Could you check a few things on this drawing? It's one solid part, dimensions in mm from its lowest x, y, z. A direction names the side the tool comes from. Coordinates: 2 decimals unless noted, no trailing zeros. Order: outer loops, then holes, each group sorted by start corner. A loop starts at its lowest first (then second) coordinate and runs counter-clockwise, first axis right, second up.
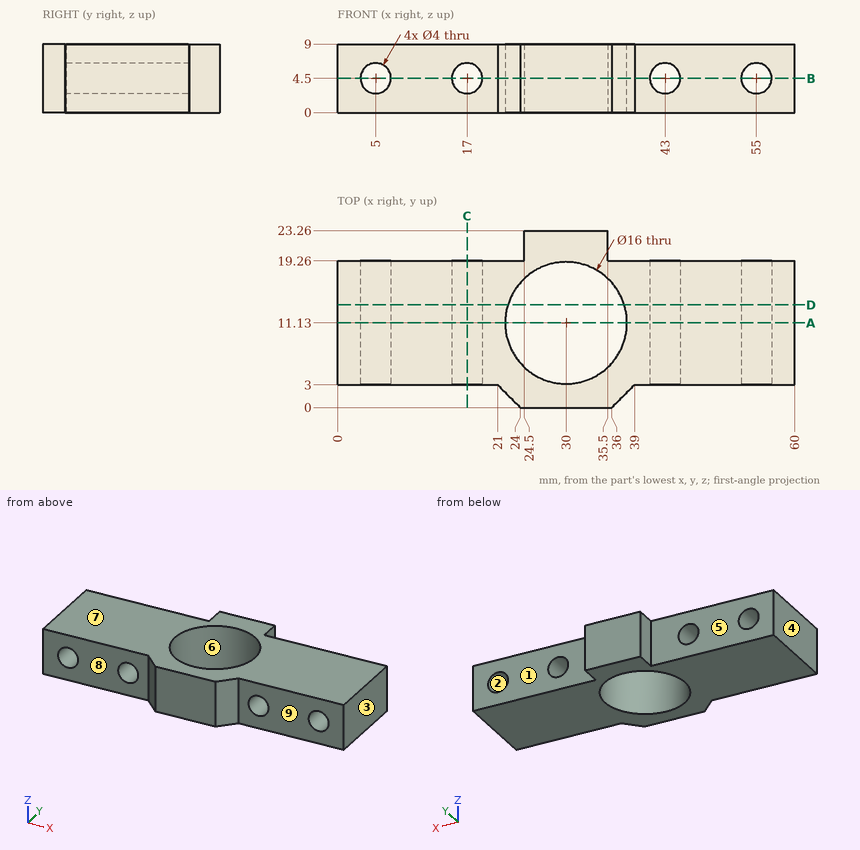
Item 1: Thinking about a two-plate mould opening in X: for the marked faces 1, 2, 3 and 4, which applies, +X half, -X half, draft (parallel to the pull), parting line (faces both ways), or undercut?
Item 2: For pin 1 Ø4 at (x, z) = (46.5, 1) entering from -Y; pin 2 Ø3 at (y, z) = (22.5, 4) entering from -X; pin 3 Ø3 at (y, z) = (21.5, 3) entering from +X; pin 4 Ø3 at (x, z) = (43, 4.5) entering from +Y, each with a flat end and sliding along its axis, tell me the tip position at first contact or that it passes through.
Item 3: Suppose I cut it at A-A (y = 11.13). List the corners of the cut face in (x, z) for me, and give its area (3 significant figures).
Item 4: Suppose I cut it at C-C (x = 17). List the corners of the cut face in (y, z) for me.
Item 5: Suppose I cut it at B-B (z = 4.5). Count the separate pieces of the cut face and the enclosed holes in it, and give its area (3 significant figures).
Item 6: Which directions (+Z, -Z, +X, -X, +Y, -Y) give clear straight access to the entire face, cutting with the end or side of a thin tool? Please do the marked faces 5, 6, 7, 8 and 9.
Item 7: I need wall thicknesses on line 1 (X direction, y = 11.25, z = 4.5); line 2 (X direction, y = 3.75, z = 2.75); line 3 (Y direction, x = 54.5, z = 1.75). Which ranges of each line are inside material? Lowest first, please.
Item 8: Suppose I cut it at D-D (y = 13.5). List the corners of the cut face in (x, z) for me, and give its area (3 significant figures).
Geometry results:
1. face 1: draft
1. face 2: undercut
1. face 3: +X half
1. face 4: -X half
2. pin 1: stops at y = 3
2. pin 2: stops at x = 24.5
2. pin 3: stops at x = 35.5
2. pin 4: passes through
3. outline: (0, 0) - (22, 0) - (22, 9) - (0, 9) - close; (38, 0) - (60, 0) - (60, 9) - (38, 9) - close; hole circle Ø4 at (5, 4.5); hole circle Ø4 at (17, 4.5); hole circle Ø4 at (43, 4.5); hole circle Ø4 at (55, 4.5)
3. area: 346 mm2
4. outline: (3, 0) - (19.26, 0) - (19.26, 2.5) - (3, 2.5) - close; (3, 6.5) - (19.26, 6.5) - (19.26, 9) - (3, 9) - close
5. separate pieces: 5
5. enclosed holes: 1
5. area: 603 mm2
6. face 5: +Z, -Z, -X, +Y
6. face 6: +Z, -Z
6. face 7: +Z, +X, -X, +Y, -Y
6. face 8: +Z, -Z, -X, -Y
6. face 9: +Z, -Z, +X, -Y
7. line 1: x = 0 to 3, 7 to 15, 19 to 22, 38 to 41, 45 to 53, 57 to 60
7. line 2: x = 0 to 4.03, 5.97 to 16.03, 17.97 to 26.91, 33.09 to 42.03, 43.97 to 54.03, 55.97 to 60
7. line 3: y = 3 to 19.26
8. outline: (0, 0) - (22.36, 0) - (22.36, 9) - (0, 9) - close; (37.64, 0) - (60, 0) - (60, 9) - (37.64, 9) - close; hole circle Ø4 at (5, 4.5); hole circle Ø4 at (17, 4.5); hole circle Ø4 at (43, 4.5); hole circle Ø4 at (55, 4.5)
8. area: 352 mm2
